```python
from build123d import *

# Parameters (mm, degrees)
SKETCH011_R     = 10
PAD005_DEPTH    = 5
FILLET_R        = 2
FILLET001_R     = 2
SKETCH012_R     = 0.75
POCKET006_DEPTH = 3.5


with BuildPart() as part:
    # Sketch011 (on Face1 of CopyPocket005) → Pad005 (new body)
    with BuildSketch(Plane.XY.offset(30)):
        with Locations((0.000374, 26)):
            Circle(SKETCH011_R)
        with BuildLine():
            ThreePointArc((-2.5, 28.5), (-5, 26), (-2.5, 23.5))
            Line((-2.5, 23.5), (2.5, 23.5))
            ThreePointArc((2.5, 23.5), (5, 26), (2.5, 28.5))
            Line((-2.5, 28.5), (2.5, 28.5))
        make_face(mode=Mode.SUBTRACT)
    extrude(amount=PAD005_DEPTH)

    # Fillet
    fillet_edges = [part.edges().sort_by_distance(p)[0] for p in [
        (-5, 26, 35),
    ]]
    fillet(fillet_edges, radius=FILLET_R)

    # Fillet001
    fillet001_edges = [part.edges().sort_by_distance(p)[0] for p in [
        (-9.999626, 26, 35),
    ]]
    fillet(fillet001_edges, radius=FILLET001_R)

    # Sketch012 (on Face12 of Fillet001) → Pocket006 (cut)
    with BuildSketch(Plane(origin=(0, 0, 30), x_dir=(1, 0, 0), z_dir=(0, 0, -1))):
        with Locations((-7.115, -26)):
            Circle(SKETCH012_R)
        with Locations((7.115, -26)):
            Circle(SKETCH012_R)
    extrude(amount=-POCKET006_DEPTH, mode=Mode.SUBTRACT)


solid = part.part
```
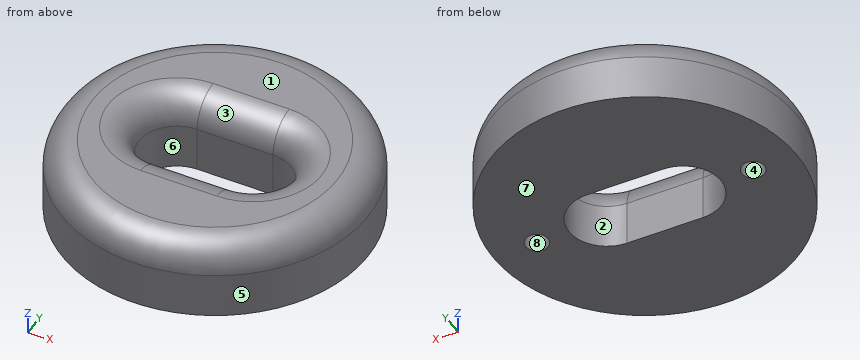
Source: CAD feature listing. Evaluate the final solid. Frame: model axes, mm. Face numbers are marked on the shaded views. A direction names the side the tool comes from. Give positions to 0.01 mm unless a question says otherwise; leave off trailing zeros. Loops run counter-clockwise (first coordinate to the right, second up) from the corner with the lowest first, then second, coordinate; pieces in that order, holes last. Notation, with made-up numbers: (8, 9) - (55, 9) arc R8 ccw to (55, 24) - close; hole circle Ø11 at (17.5, 85.5). An arc over 180 degrees is marked (long way). Use CSV: the item, a comma, the result in double quotes.
1) Set-up query: the marked faces 1, 2, 3 and 4. Return all of +Z, -Z, +X, -X, +Y, -Y with unobstructed straight access to the full face (end or side cutting, diameter ignored); none if empty.
Worked out:
face 1,"+Z, +X, -X, +Y, -Y"
face 2,"+Z, -Z"
face 3,"+Z"
face 4,"-Z"
2) Mould query, pull axis X, two halves, no side actions, for the marked faces 5, 6, 7 and 8. Classes: +X half, -X half, draft (parallel to the pull), parting line (faces both ways), or undercut.
Worked out:
face 5,"parting line"
face 6,"undercut"
face 7,"draft"
face 8,"undercut"
3) Pin query (flat end, axial travel): P1, Ø1.5, axis at y = 24.5, z = 32, coming from the +X side; P2, Ø0.8, axis at x = -7, y = 26, coming from the -Z side; P3, Ø1, axis at x = 3, z = 33.5, coming from the -Y side. Return the tip coordinate at first contact, or that it passes through.
Worked out:
P1,"stops at x = 9.97"
P2,"stops at z = 33.5"
P3,"stops at y = 16.35"
4) Line query: line 1 (Y direction, x = -0.25, z = 31.55); line 2 (X direction, y = 26.5, z = 30.8); line 3 (Y direction, x = 4, z = 34.5). Output: solid intervals per line, ascending.
Worked out:
line 1,"y = 16 to 23.5, 28.5 to 36"
line 2,"x = -9.99 to -7.67, -6.56 to -4.95, 4.95 to 6.56, 7.67 to 9.99"
line 3,"y = 17.58 to 23.2, 28.8 to 34.42"
5) Cut plane C-C (z = 33.85). Output: boundary loops of the cut face in (x, y).
Worked out:
outline,"circle Ø19.62 at (0, 26); hole (-2.5, 23.31) - (2.5, 23.31) arc R2.69 ccw to (2.5, 28.69) - (-2.5, 28.69) arc R2.69 ccw to start"
6) Cut plane B-B (z = 30.5). Output: boundary loops of the cut face in (x, y) (3 decimals).
Worked out:
outline,"circle Ø20 at (0, 26); hole circle Ø1.5 at (-7.115, 26); hole (-2.5, 23.5) - (2.5, 23.5) arc R2.5 ccw to (2.5, 28.5) - (-2.5, 28.5) arc R2.5 ccw to start; hole circle Ø1.5 at (7.115, 26)"
7) Cut plane A-A (y = 26). Output: boundary loops of the cut face in (x, z) (3 decimals).
Worked out:
outline,"(-10, 30) - (-7.865, 30) - (-7.865, 33.5) - (-6.365, 33.5) - (-6.365, 30) - (-5, 30) - (-5, 33) arc R2 ccw to (-7, 35) - (-8, 35) arc R2 ccw to (-10, 33) - close; (5, 30) - (6.365, 30) - (6.365, 33.5) - (7.865, 33.5) - (7.865, 30) - (10, 30) - (10, 33) arc R2 ccw to (8, 35) - (7, 35) arc R2 ccw to (5, 33) - close"
